from build123d import *

# Parameters (mm, degrees)
SKETCH1_W           = 61.8
SKETCH1_H           = 62
BOSS_EXTRUDE1_DEPTH = 3.2
CUT_EXTRUDE1_REACH  = 5.2
SKETCH2_R           = 21.05
CUT_EXTRUDE2_REACH  = 5.2
SKETCH3_R           = 2.625


with BuildPart() as part:
    # Sketch1 → Boss-Extrude1 (new body)
    with BuildSketch(Plane(origin=(0, 0, 0), x_dir=(0, 0, -1), z_dir=(1, 0, 0))):
        with Locations((30.9, 31)):
            Rectangle(SKETCH1_W, SKETCH1_H)
    extrude(amount=BOSS_EXTRUDE1_DEPTH)

    # Sketch2 → Cut-Extrude1 (cut, up to next)
    with BuildSketch(Plane(origin=(3.2, 0, 0), x_dir=(0, 0, -1), z_dir=(1, 0, 0)), mode=Mode.PRIVATE) as cut_extrude1_sk1:
        with Locations((30.9, 32)):
            Circle(SKETCH2_R)
    cut_extrude1_tool1 = extrude(cut_extrude1_sk1.sketch, amount=-CUT_EXTRUDE1_REACH, mode=Mode.PRIVATE) & part.part
    add(cut_extrude1_tool1.solids().sort_by_distance((3.2, 32, -30.9))[0], mode=Mode.SUBTRACT)

    # Sketch3 → Cut-Extrude2 (cut, up to next)
    with BuildSketch(Plane.ZY, mode=Mode.PRIVATE) as cut_extrude2_sk1:
        with Locations((-54.3, 49)):
            Circle(SKETCH3_R)
    cut_extrude2_tool1 = extrude(cut_extrude2_sk1.sketch, amount=-CUT_EXTRUDE2_REACH, mode=Mode.PRIVATE) & part.part
    add(cut_extrude2_tool1.solids().sort_by_distance((0, 49, -54.3))[0], mode=Mode.SUBTRACT)
    # Sketch3 → Cut-Extrude2 (cut, up to next)
    with BuildSketch(Plane.ZY, mode=Mode.PRIVATE) as cut_extrude2_sk2:
        with Locations((-54.3, 13)):
            Circle(SKETCH3_R)
    cut_extrude2_tool2 = extrude(cut_extrude2_sk2.sketch, amount=-CUT_EXTRUDE2_REACH, mode=Mode.PRIVATE) & part.part
    add(cut_extrude2_tool2.solids().sort_by_distance((0, 13, -54.3))[0], mode=Mode.SUBTRACT)
    # Sketch3 → Cut-Extrude2 (cut, up to next)
    with BuildSketch(Plane.ZY, mode=Mode.PRIVATE) as cut_extrude2_sk3:
        with Locations((-7.5, 49)):
            Circle(SKETCH3_R)
    cut_extrude2_tool3 = extrude(cut_extrude2_sk3.sketch, amount=-CUT_EXTRUDE2_REACH, mode=Mode.PRIVATE) & part.part
    add(cut_extrude2_tool3.solids().sort_by_distance((0, 49, -7.5))[0], mode=Mode.SUBTRACT)
    # Sketch3 → Cut-Extrude2 (cut, up to next)
    with BuildSketch(Plane.ZY, mode=Mode.PRIVATE) as cut_extrude2_sk4:
        with Locations((-7.5, 13)):
            Circle(SKETCH3_R)
    cut_extrude2_tool4 = extrude(cut_extrude2_sk4.sketch, amount=-CUT_EXTRUDE2_REACH, mode=Mode.PRIVATE) & part.part
    add(cut_extrude2_tool4.solids().sort_by_distance((0, 13, -7.5))[0], mode=Mode.SUBTRACT)


solid = part.part
The model under review builds one solid part; all positions refer to its coordinate system, in mm. Coordinates: 2 decimals unless noted, no trailing zeros. Write each loop counter-clockwise with the first axis right and the second up, starting at its lowest first coordinate (ties: lowest second). Pieces come first, ordered by that corner, then holes. Notation, with made-up numbers: (13, -13.5) - (70, -13.5) arc R31 ccw to (70, 20.5) - close; hole circle Ø3 at (56, 24). An arc over 180 degrees is marked (long way). Answer as CSV lines item,"result".
(1) Clearance check with a flat-ended pin moving along its axis: pin 1 Ø7 at (y, z) = (13, -54.3) entering from -X. State where the tip first meets the part, or that it passes through.
Data:
pin 1,"stops at x = 0"
(2) We need section A-A (z = -30.9). Give the boundary of the cut face in (x, y), plus the area to 3 significant figures.
Data:
outline,"(0, 0) - (3.2, 0) - (3.2, 10.95) - (0, 10.95) - close; (0, 53.05) - (3.2, 53.05) - (3.2, 62) - (0, 62) - close"
area,"63.7 mm2"
(3) Mouldability with a two-part tool opening along Y and no side actions: class faces 1 (the cylindrical face through (1.578, 49.115, -56.922)), 2 (the flat face through (2, 0, -30)), 3 (the flat face through (2, 31, -61.8)) as pulls with the +Y half, pulls with the -Y half, needs draft (parallel to the pull), parting line crosses it, or undercut.
Data:
face 1,"undercut"
face 2,"pulls with the -Y half"
face 3,"needs draft"
(4) For line 1 along Y through (x, z) = (2.15, -54.3) (3 decimals); line 2 along Y through (x, z) = (1.5, -30.9); line 3 along Z through (x, y) = (1.35, 13.5), list the stretches that pass through material, from the lowest coordinate up. Write a range as [from, to].
Data:
line 1,"y = [0, 10.375], [15.625, 46.375], [51.625, 62]"
line 2,"y = [0, 10.95], [53.05, 62]"
line 3,"z = [-61.8, -56.88], [-51.72, -40.94], [-20.86, -10.08], [-4.92, 0]"
(5) We need section D-D (z = -7.5). Give the boundary of the cut face in (x, y) (3 decimals).
Data:
outline,"(0, 0) - (3.2, 0) - (3.2, 10.375) - (0, 10.375) - close; (0, 15.625) - (3.2, 15.625) - (3.2, 46.375) - (0, 46.375) - close; (0, 51.625) - (3.2, 51.625) - (3.2, 62) - (0, 62) - close"
(6) We need section C-C (x = 2.6). Give the boundary of the cut face in (y, z) (3 decimals), plus the area to 3 significant figures.
Data:
outline,"(0, -61.8) - (62, -61.8) - (62, 0) - (0, 0) - close; hole circle Ø5.25 at (13, -54.3); hole circle Ø5.25 at (13, -7.5); hole circle Ø42.1 at (32, -30.9); hole circle Ø5.25 at (49, -54.3); hole circle Ø5.25 at (49, -7.5)"
area,"2,350 mm2"
(7) We need section B-B (y = 32). Give the boundary of the cut face in (x, z), plus the area to 3 significant figures.
Data:
outline,"(0, -61.8) - (3.2, -61.8) - (3.2, -51.95) - (0, -51.95) - close; (0, -9.85) - (3.2, -9.85) - (3.2, 0) - (0, 0) - close"
area,"63.0 mm2"
